Design review of the part built by this model. Coordinates are the model's own, in mm. Face numbers are marked on the shaded views. A direction names the side the tool comes from. Round coordinates to 2 decimals unless told otherwise and drop trailing zeros. Write each loop counter-clockwise with the first axis right and the second up, starting at its lowest first coordinate (ties: lowest second). Pieces come first, ordered by that corner, then holes. Notation, with made-up numbers: (-10.5, -4.75) - (27.5, -4.75) arc R9 ccw to (27.5, 1.25) - close; hole circle Ø6 at (-34.5, 54.5). An arc over 180 degrees is marked (long way). Use one line per item in the form item = value.
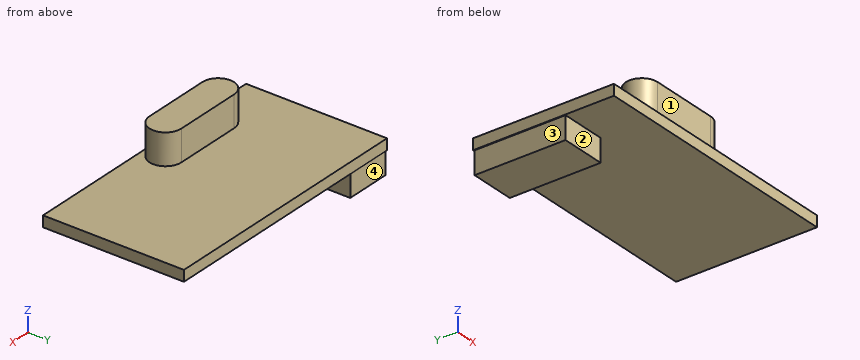
```python
from build123d import *

# Parameters (mm, degrees)
BOSS_EXTRUDE1_DEPTH = 1.2
BOSS_EXTRUDE2_DEPTH = 3.4
SKETCH3_W           = 5
SKETCH3_H           = 10
BOSS_EXTRUDE3_DEPTH = 2.5


with BuildPart() as part:
    # Sketch1 → Boss-Extrude1 (new body)
    with BuildSketch(Plane.XY):
        Polygon((-14.45, 7.75), (14.45, 7.75), (-14.45, -7.75), align=None)
        Polygon((14.45, 7.75), (14.45, -7.75), (-14.45, -7.75), align=None)
    extrude(amount=BOSS_EXTRUDE1_DEPTH)

    # Sketch2 → Boss-Extrude2 (add)
    with BuildSketch(Plane.XY.offset(1.2)):
        with BuildLine():
            Line((-7.7, -3.85), (-0.2, -3.85))
            ThreePointArc((-0.2, -3.85), (1.55, -5.6), (-0.2, -7.35))
            Line((-0.2, -7.35), (-7.7, -7.35))
            ThreePointArc((-7.7, -7.35), (-9.45, -5.6), (-7.7, -3.85))
        make_face()
    extrude(amount=BOSS_EXTRUDE2_DEPTH)

    # Sketch3 → Boss-Extrude3 (add)
    with BuildSketch(Plane(origin=(0, 0, 0), x_dir=(-1, 0, 0), z_dir=(0, 0, -1))):
        with Locations((11.85, 2.65)):
            Rectangle(SKETCH3_W, SKETCH3_H)
    extrude(amount=BOSS_EXTRUDE3_DEPTH)


solid = part.part
```
Q1. To check wall thickness, follow line 1 along Z through (x, y) = (-1, 3.5); line 2 along Y through (x, z) = (-4.25, 2.25); line 3 along Z through (x, y) = (-1, -7). State the ranges of each line that lie inside material, in increasing order. Write a range as from..to.
Calculated:
line_1 = 0..1.2
line_2 = -7.35..-3.85
line_3 = 0..4.6
Q2. We need section A-A on y = 2.75. Write out the cut boundary in (x, z), then the cut area to 3 significant figures.
Calculated:
outline = (-14.45, 0) - (-14.35, 0) - (-14.35, -2.5) - (-9.35, -2.5) - (-9.35, 0) - (14.45, 0) - (14.45, 1.2) - (-14.45, 1.2) - close
area = 47.2 mm2
Q3. Machinability: for the marked faces 1, 2, 3 and 4, which of the approach directions +Z, -Z, +X, -X, +Y, -Y give a long, thin tool a straight path to every point of the face, cutting with its end or side? Answer none if there is none.
Calculated:
face_1 = +Z, +X, -X, -Y
face_2 = -Z, +X, -X, -Y
face_3 = -Z, -X, +Y, -Y
face_4 = -Z, +X, -X, +Y
Q4. We need section C-C on z = 1.75. Write out the cut boundary in (x, y), then the cut area to 3 significant figures.
Calculated:
outline = (-7.7, -7.35) - (-0.2, -7.35) arc R1.75 ccw to (-0.2, -3.85) - (-7.7, -3.85) arc R1.75 ccw to start
area = 35.9 mm2
Q5. We need section B-B on x = -11.75. Write out the cut boundary in (y, z).
Calculated:
outline = (-7.75, 0) - (-2.35, 0) - (-2.35, -2.5) - (7.65, -2.5) - (7.65, 0) - (7.75, 0) - (7.75, 1.2) - (-7.75, 1.2) - close
Q6. We need section D-D on x = 8.25. Write out the cut boundary in (y, z), then the cut area to 3 significant figures.
Calculated:
outline = (-7.75, 0) - (7.75, 0) - (7.75, 1.2) - (-7.75, 1.2) - close
area = 18.6 mm2
Q7. For P1, Ø4, axis at x = -7, y = 1.5, coming from the -Z side; P2, Ø1.2, axis at y = 0.5, z = -0.5, coming from the -X side; P3, Ø1, axis at x = 11, z = -1, coming from the +Y side; P4, Ø2.5, axis at x = -5, z = 2.5, coming from the +Y side, all flat-tipped, find the tip position at first contact; note any pin that passes through.
Calculated:
P1 = 0
P2 = -14.45
P3 = through
P4 = -3.85
